Could you check a few things on this model? Use its own coordinates, in mm. Round coordinates to 2 decimals unless told otherwise and drop trailing zeros. Write each loop counter-clockwise with the first axis right and the second up, starting at its lowest first coordinate (ties: lowest second). Pieces come first, ordered by that corner, then holes. Notation, with made-up numbers: M 47,37.5 L 99,37.5 A22 cw 99,52.5 Z; hole C -13,72 d7. An arc over 180 degrees is marked long. One line per item, written item: value. Start each with the question number.
(1) If I drill on L1, parallel to X at y = 3.95, z = 21; L2, parallel to X at y = 0.35, z = -2; L3, parallel to X at y = 4.65, z = -19.5, over which ranges is the centre line in solid material (lowest first)?
(2) I want a section at D-D on z = -15. Please give me the cut outline in (x, y), and give its area (3 significant figures).
(3) I want a section at C-C on x = -9. Please give me the cut outline in (y, z), and give its area (3 significant figures).
(4) I want a section at B-B on z = 0. Please give me the cut outline in (x, y), and give its area (3 significant figures).
(5) I want a section at A-A on x = 0. Please give me the cut outline in (y, z), and give its area (3 significant figures).
(6) I'm going to push flat-ended pins straight in: pin 1 Ø8 at (x, z) = (3, -15) entering from -Y; pin 2 Ø3 at (y, z) = (2, 15) entering from -X; pin 3 Ø2 at (x, y) = (21, 1) entering from +Z; pin 4 Ø3 at (y, z) = (3.5, 24) entering from +X. Where does each tip first touch, or does it pass through?
Autodesk Inventor part; units mm, degrees
ref_plane "YZ Plane" through (0, 0, 0) normal (1, 0, 0) x (0, 1, 0)
ref_plane "XZ Plane" through (0, 0, 0) normal (0, 1, 0) x (-1, 0, 0)
ref_plane "XY Plane" through (0, 0, 0) normal (0, 0, 1) x (1, 0, 0)
sketch "스케치1" plane through (0, 0, 0) normal (0, 1, 0) x (-1, 0, 0)
  circle A0 centre (0, 0) radius 35
  circle A1 centre (0, 0) radius 7.5
  circle A2 centre (0, 0) radius 12.5
  circle A3 centre (0, 0) radius 30
  dimension "d0" = 70
  dimension "d1" = 15
  dimension "d2" = 25
  dimension "d3" = 60
extrude "돌출1" add sketch "스케치1" along normal blind 5
sketch "스케치2" plane through (0, 0, 0) normal (0, -1, 0) x (1, 0, 0)
  line L0 (-10.8253, 6.25) -> (-25.9808, 15)
  circle A0 centre (0, 0) radius 30
  circle A1 centre (0, 0) radius 7.5
  circle A2 centre (0, 0) radius 7.5
  circle A3 centre (0, 0) radius 12.5
  circle A4 centre (0, 0) radius 12.5
  line L1 (0, 12.5) -> (0, 30)
  line L2 (10.8253, 6.25) -> (25.9808, 15)
  line L3 (10.8253, -6.25) -> (25.9808, -15)
  line L4 (0, -12.5) -> (0, -30)
  line L5 (-10.8253, -6.25) -> (-25.9808, -15)
  line L6 (-1.5, 34.9678) -> (1.5, 34.9678)
  line L7 (1.5, 34.9678) -> (1.5, 12.4097)
  line L8 (1.5, 12.4097) -> (-1.5, 12.4097)
  line L9 (-1.5, 12.4097) -> (-1.5, 34.9678)
  circle A5 centre (0, 0) radius 35
  dimension "d10" = 3
  dimension "d11" = 1.5
extrude "돌출2" add sketch "스케치2" against normal blind 5 contours L9 A0 L1 A3 | L9 L6 L7 A0 | L1 A0 L7 A3
pattern_circular "원형 패턴1" count 6 over 360 about axis through (0, 0, 0) along (0, 1, 0) of "돌출2"
properties part number "부품2"
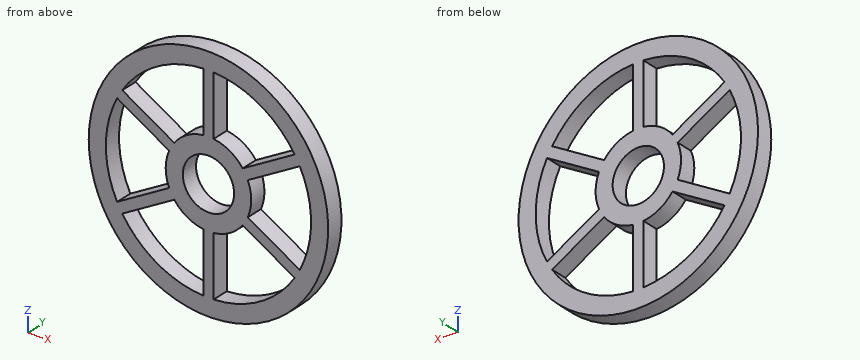
Found:
1. L1: x = -28 to -21.42, -1.5 to 1.5, 21.42 to 28
1. L2: x = -34.94 to -29.93, -12.34 to -7.23, 7.23 to 12.34, 29.93 to 34.94
1. L3: x = -29.06 to -22.8, -1.5 to 1.5, 22.8 to 29.06
2. outline: M -31.62,0 L -22.98,0 L -22.98,5 L -31.62,5 Z; M -1.5,0 L 1.5,0 L 1.5,5 L -1.5,5 Z; M 22.98,0 L 31.62,0 L 31.62,5 L 22.98,5 Z
2. area: 101 mm²
3. outline: M 0,-33.82 L 5,-33.82 L 5,-28.62 L 0,-28.62 Z; M 0,-8.67 L 5,-8.67 L 5,8.67 L 0,8.67 Z; M 0,28.62 L 5,28.62 L 5,33.82 L 0,33.82 Z
3. area: 139 mm²
4. outline: M -35,0 L -30,0 L -30,5 L -35,5 Z; M -12.5,0 L -7.5,0 L -7.5,5 L -12.5,5 Z; M 7.5,0 L 12.5,0 L 12.5,5 L 7.5,5 Z; M 30,0 L 35,0 L 35,5 L 30,5 Z
4. area: 100 mm²
5. outline: M 0,-35 L 5,-35 L 5,-7.5 L 0,-7.5 Z; M 0,7.5 L 5,7.5 L 5,35 L 0,35 Z
5. area: 275 mm²
6. pin 1: stops at y = 0
6. pin 2: stops at x = -32.29
6. pin 3: stops at z = 28.72
6. pin 4: stops at x = 26.81
